Could you check a few things on this model? Use its own coordinates, in mm. Give positions to 0.01 mm unless a question says otherwise; leave off trailing zeros.
from build123d import *

# Parameters (mm, degrees)
SKETCH1_W           = 146
SKETCH1_H           = 100
BOSS_EXTRUDE1_DEPTH = 3
SKETCH2_W           = 1
SKETCH2_H           = 45
CUT_EXTRUDE1_DEPTH  = 4
SKETCH3_R           = 2
CUT_EXTRUDE2_DEPTH  = 4
SKETCH4_W           = 11.62
SKETCH4_H           = 9
CUT_EXTRUDE3_DEPTH  = 4
SKETCH5_W           = 14.16
SKETCH5_H           = 9
CUT_EXTRUDE4_DEPTH  = 4
SKETCH6_R           = 3.5
CUT_EXTRUDE5_DEPTH  = 4
SKETCH8_R           = 2
CUT_EXTRUDE6_DEPTH  = 4
SKETCH9_R           = 2
CUT_EXTRUDE7_DEPTH  = 4


with BuildPart() as part:
    # Sketch1 → Boss-Extrude1 (new body)
    with BuildSketch(Plane.XY):
        with Locations((24.755849622, 29.633412311)):
            Rectangle(SKETCH1_W, SKETCH1_H)
    extrude(amount=BOSS_EXTRUDE1_DEPTH)

    # Sketch2 → Cut-Extrude1 (cut, through all)
    with BuildSketch(Plane.XY.offset(3)):
        with Locations((-19.744150378, 32.133412311)):
            Rectangle(SKETCH2_W, SKETCH2_H)
        with Locations((-25.744150378, 32.133412311)):
            Rectangle(SKETCH2_W, SKETCH2_H)
        with Locations((-13.744150378, 32.133412311)):
            Rectangle(SKETCH2_W, SKETCH2_H)
        with Locations((-7.744150378, 32.133412311)):
            Rectangle(SKETCH2_W, SKETCH2_H)
        with Locations((-1.744150378, 32.133412311)):
            Rectangle(SKETCH2_W, SKETCH2_H)
        with Locations((4.255849622, 32.133412311)):
            Rectangle(SKETCH2_W, SKETCH2_H)
        with Locations((10.255849622, 32.133412311)):
            Rectangle(SKETCH2_W, SKETCH2_H)
        with Locations((16.255849622, 32.133412311)):
            Rectangle(SKETCH2_W, SKETCH2_H)
        with Locations((22.255849622, 32.133412311)):
            Rectangle(SKETCH2_W, SKETCH2_H)
        with Locations((34.255849622, 32.133412311)):
            Rectangle(SKETCH2_W, SKETCH2_H)
        with Locations((28.255849622, 32.133412311)):
            Rectangle(SKETCH2_W, SKETCH2_H)
        with Locations((40.255849622, 32.133412311)):
            Rectangle(SKETCH2_W, SKETCH2_H)
        with Locations((46.255849622, 32.133412311)):
            Rectangle(SKETCH2_W, SKETCH2_H)
        with Locations((52.255849622, 32.133412311)):
            Rectangle(SKETCH2_W, SKETCH2_H)
        with Locations((58.255849622, 32.133412311)):
            Rectangle(SKETCH2_W, SKETCH2_H)
        with Locations((64.255849622, 32.133412311)):
            Rectangle(SKETCH2_W, SKETCH2_H)
        with Locations((70.255849622, 32.133412311)):
            Rectangle(SKETCH2_W, SKETCH2_H)
        with Locations((76.255849622, 32.133412311)):
            Rectangle(SKETCH2_W, SKETCH2_H)
    extrude(amount=-CUT_EXTRUDE1_DEPTH, mode=Mode.SUBTRACT)

    # Sketch3 → Cut-Extrude2 (cut, through all)
    with BuildSketch(Plane.XY.offset(3)):
        with Locations((-33.244150378, -5.366587689)):
            Circle(SKETCH3_R)
        with Locations((82.755849622, -5.366587689)):
            Circle(SKETCH3_R)
    extrude(amount=-CUT_EXTRUDE2_DEPTH, mode=Mode.SUBTRACT)

    # Sketch4 → Cut-Extrude3 (cut, through all)
    with BuildSketch(Plane(origin=(0, 0, 0), x_dir=(-1, 0, 0), z_dir=(0, 0, -1))):
        with Locations((-47.025849622, -8.521305626)):
            Rectangle(SKETCH4_W, SKETCH4_H)
    extrude(amount=-CUT_EXTRUDE3_DEPTH, mode=Mode.SUBTRACT)

    # Sketch5 → Cut-Extrude4 (cut, through all)
    with BuildSketch(Plane.XY.offset(3)):
        with Locations((26.385849622, -8.521305626)):
            Rectangle(SKETCH5_W, SKETCH5_H)
    extrude(amount=-CUT_EXTRUDE4_DEPTH, mode=Mode.SUBTRACT)

    # Sketch6 → Cut-Extrude5 (cut, through all)
    with BuildSketch(Plane(origin=(0, 0, 0), x_dir=(-1, 0, 0), z_dir=(0, 0, -1))):
        with Locations((-9.139177798, -4.021305626)):
            Circle(SKETCH6_R)
        with Locations((5.860822202, -4.021305626)):
            Circle(SKETCH6_R)
    extrude(amount=-CUT_EXTRUDE5_DEPTH, mode=Mode.SUBTRACT)

    # Sketch8 → Cut-Extrude6 (cut, through all)
    with BuildSketch(Plane.XY.offset(3)):
        with Locations((82.755849622, 24.633412311)):
            Circle(SKETCH8_R)
        with Locations((-33.244150378, 24.633412311)):
            Circle(SKETCH8_R)
    extrude(amount=-CUT_EXTRUDE6_DEPTH, mode=Mode.SUBTRACT)

    # Sketch9 → Cut-Extrude7 (cut, through all)
    with BuildSketch(Plane.XY.offset(3)):
        with Locations((-21.244150378, 64.633412311)):
            Circle(SKETCH9_R)
        with Locations((70.77306316, 61.532054099)):
            Circle(SKETCH9_R)
    extrude(amount=-CUT_EXTRUDE7_DEPTH, mode=Mode.SUBTRACT)


solid = part.part
Item 1: Please list where these lines run through material, in increasing order: line 1 along X through (y, z) = (-8.5, 1.9); line 2 along Y through (x, z) = (43, 0.85); line 3 along Y through (x, z) = (34, 1.6).
Findings:
line 1: x = -48.24 to 19.31, 33.47 to 41.22, 52.84 to 97.76
line 2: y = -20.37 to -13.02, -4.02 to 79.63
line 3: y = -20.37 to 9.63, 54.63 to 79.63
Item 2: We'd pull the mould along Y, two halves only. Please class faces 1 (the flat face through (97.756, 29, 1)), 2 (the flat face through (10.756, 32, 2)): +Y half, -Y half, draft (parallel to the pull), parting line (faces both ways), or undercut.
Findings:
face 1: draft
face 2: undercut
Item 3: Imagine slicing it at A-A on y = 36. Give the number of separate pieces and of enclosed holes in the cut face, then the cut area to 3 significant figures.
Findings:
separate pieces: 19
enclosed holes: 0
area: 384 mm2
